Geometry check sheet. Reference: the model listing, model coordinates, mm. Face numbers are marked on the shaded views. A direction names the side the tool comes from. Round coordinates to 2 decimals unless told otherwise and drop trailing zeros. Order: outer loops, then holes, each group sorted by start corner. A loop starts at its lowest first (then second) coordinate and runs counter-clockwise, first axis right, second up.
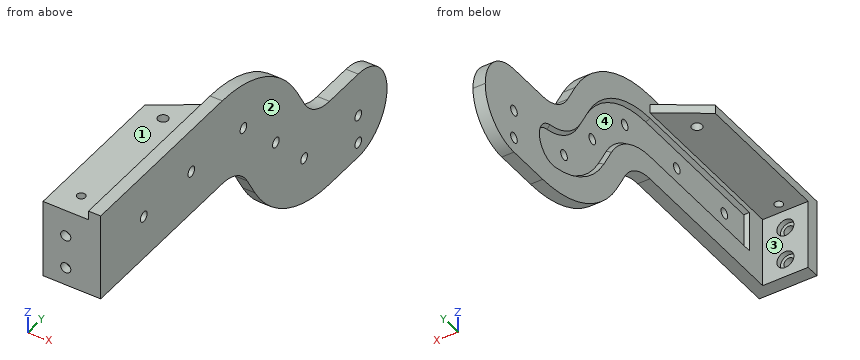
```python
from build123d import *

# Parameters (mm, degrees)
SKETCH_2_W                = 3.6
SKETCH_2_H                = 26
SKETCH_3_W                = 17
SKETCH_3_H                = 33
EXTRUDE_1_DEPTH           = 4
RIB_START                 = -1.3
RIB_1_DEPTH               = 2.6
SKETCH_5_R                = 1.5
SKETCH_5_R_2              = 1.224086187
CUT_EXTRUDE_1_DEPTH       = 4
CUT_EXTRUDE_2_DEPTH       = 4
SKETCH_7_R                = 1.5
CUT_EXTRUDE_3_DEPTH       = 4
CUT_EXTRUDE_4_DEPTH       = 1.2
CUT_EXTRUDE_4_DRAFT       = -30
HOLE_WIZARD_1_D           = 3
HOLE_WIZARD_1_CBORE_D     = 5
HOLE_WIZARD_1_CBORE_DEPTH = 1.6
CUT_EXTRUDE_6_DEPTH       = 135.185107528
SKETCH_25_R               = 1.5
CUT_EXTRUDE_8_DEPTH       = 139.143340278


# Read off the part's stored shape, not the designer's step: 筋1
with BuildPart() as part:
    # 扫描1: sweep along a path in 草图1
    with BuildLine(Plane(origin=(0, 0, 0), x_dir=(0, 0, -1), z_dir=(1, 0, 0))) as sweep_1_path:
        Line((0, 0), (0, 55))
        ThreePointArc((0, 55), (3.483339502, 68), (13, 77.516660498))
        Line((13, 77.516660498), (19, 80.980762114))
        ThreePointArc((19, 80.980762114), (28.516660498, 90.497422612), (32, 103.497422612))
        Line((32, 103.497422612), (32, 129.497422612))
    # 草图2 → 扫描1 (sweep)
    with BuildSketch(Plane(origin=(0, 0, 0), x_dir=(1, 0, 0), z_dir=(0, 1, 0))):
        Rectangle(SKETCH_2_W, SKETCH_2_H)
    sweep(path=sweep_1_path.line)

    # 草图3 → 凸台-拉伸1 (add)
    with BuildSketch(Plane.XZ):
        with Locations((-6.7, 3.5)):
            Rectangle(SKETCH_3_W, SKETCH_3_H)
    extrude(amount=-EXTRUDE_1_DEPTH)

    # 筋1 outline → 筋1 (add)
    with BuildSketch(Plane.XY.offset(9).offset(RIB_START)):
        Polygon((-1.8, 55), (-15.2, 46), (-15.2, 4), (-1.8, 4), align=None)
    extrude(amount=RIB_1_DEPTH)

    # 草图5 → 切除-拉伸1 (cut)
    with BuildSketch(Plane.XY.offset(10.3)):
        with Locations((-8.5, 44)):
            Circle(SKETCH_5_R)
        with Locations((-8.5, 7)):
            Circle(SKETCH_5_R_2)
    extrude(amount=-CUT_EXTRUDE_1_DEPTH, mode=Mode.SUBTRACT)

    # 草图6 → 切除-拉伸2 (cut)
    with BuildSketch(Plane.ZY.offset(1.8)):
        with BuildLine():
            Line((-45, 129.497422612), (-45, 116.497422612))
            ThreePointArc((-45, 116.497422612), (-41.192388155, 125.689810767), (-32, 129.497422612))
            Line((-32, 129.497422612), (-45, 129.497422612))
        make_face()
        with BuildLine():
            ThreePointArc((-32, 129.497422612), (-22.807611845, 125.689810767), (-19, 116.497422612))
            Line((-19, 116.497422612), (-19, 129.497422612))
            Line((-19, 129.497422612), (-32, 129.497422612))
        make_face()
    extrude(amount=-CUT_EXTRUDE_2_DEPTH, mode=Mode.SUBTRACT)

    # 草图7 → 切除-拉伸3 (cut)
    with BuildSketch(Plane(origin=(1.8, 0, 0), x_dir=(0, 0, -1), z_dir=(1, 0, 0))):
        with Locations((32, 116.497422612)):
            Circle(SKETCH_7_R)
        with Locations((40.5, 116.497422612)):
            Circle(SKETCH_7_R)
    extrude(amount=-CUT_EXTRUDE_3_DEPTH, mode=Mode.SUBTRACT)


with BuildPart() as cut_extrude_4_tool:
    # 草图8 → 切除-拉伸4 (with draft: the straight prism first)
    with BuildSketch(Plane.ZY.offset(1.8)):
        with BuildLine():
            Line((6, 10), (6, 55))
            ThreePointArc((6, 55), (1.712812921, 71), (-10, 82.712812921))
            Line((-10, 82.712812921), (-16, 86.176914536))
            ThreePointArc((-16, 86.176914536), (-22.383040886, 92.025893885), (-25.69615506, 100.024459059))
            ThreePointArc((-25.69615506, 100.024459059), (-32.646890644, 104.891416511), (-37.513848096, 97.940680927))
            ThreePointArc((-37.513848096, 97.940680927), (-32.212865417, 85.142976649), (-22, 75.784609691))
            Line((-22, 75.784609691), (-16, 72.320508076))
            ThreePointArc((-16, 72.320508076), (-8.679491924, 65), (-6, 55))
            Line((-6, 55), (-6, 10))
            Line((-6, 10), (6, 10))
        make_face()
    extrude(amount=-CUT_EXTRUDE_4_DEPTH)
    # 切除-拉伸4: the draft: its side faces are tilted about the plane it starts from
    cut_extrude_4_sides = [cut_extrude_4_tool.faces().sort_by_distance(p)[0] for p in [
        (-1.2, 32.5, 6),
        (-1.2, 71, 1.712812921),
        (-1.2, 84.444863729, -13),
        (-1.2, 92.025893885, -22.383040886),
        (-1.2, 104.891416511, -32.646890644),
        (-1.2, 85.142976649, -32.212865417),
        (-1.2, 74.052558883, -19),
        (-1.2, 65, -8.679491924),
        (-1.2, 32.5, -6),
        (-1.2, 10, 0),
    ]]
    draft(cut_extrude_4_sides, Plane.ZY.offset(1.8), CUT_EXTRUDE_4_DRAFT)


with BuildPart() as part_1:
    add(part.part)

    # 切除-拉伸4: cut by cut_extrude_4_tool
    add(cut_extrude_4_tool.part, mode=Mode.SUBTRACT)

    # 孔1 (through all)
    with Locations(Plane(origin=(0, 4, 0), x_dir=(1, 0, 0), z_dir=(0, 1, 0))):
        with Locations((-8.5, 7.65), (-8.5, -2.35)):
            CounterBoreHole(HOLE_WIZARD_1_D / 2, HOLE_WIZARD_1_CBORE_D / 2, HOLE_WIZARD_1_CBORE_DEPTH)

    # 草图18 → 切除-拉伸6 (cut, through all)
    with BuildSketch(Plane(origin=(0, 4, 0), x_dir=(1, 0, 0), z_dir=(0, 1, 0))):
        Polygon((-1.8, -13), (-1.8, -10.3), (-15.2, -10.3), (-15.2, -20), (1.8, -20), (1.8, -13), align=None)
    extrude(amount=-CUT_EXTRUDE_6_DEPTH, mode=Mode.SUBTRACT)

    # 草图25 → 切除-拉伸8 (cut, through all)
    with BuildSketch(Plane(origin=(1.8, 0, 0), x_dir=(0, 0, -1), z_dir=(1, 0, 0))):
        with Locations((0, 19.490691587)):
            Circle(SKETCH_25_R)
    cut_extrude_8 = extrude(amount=-CUT_EXTRUDE_8_DEPTH, mode=Mode.SUBTRACT)

    # 草图阵列1: 切除-拉伸8 at 4 more places
    with Locations((0, 21.499351, 0), (0, 45.068964, -1.821229), (0, 72.524124, -29.327017), (0, 59.75802, -16)):
        add(cut_extrude_8, mode=Mode.SUBTRACT)


solid = part_1.part
```
(1) Depth check by flat-ended pin: P1, Ø4, axis at x = -9, z = 3, coming from the +Y side; P2, Ø4, axis at x = -8.5, z = -7.65, coming from the -Y side; P3, Ø8.5, axis at x = -9.5, y = 39, coming from the -Z side; P4, Ø6.5, axis at x = -9, y = 33, coming from the +Z side. Enter the tip coordinate at first touch or a pass-through.
Returned:
P1: stops at y = 4
P2: stops at y = 0
P3: stops at z = 7.7
P4: stops at z = 10.3
(2) Sectioned sample at B-B, the plane x = -8.5. Give the number of separate pieces and of enclosed holes in the cut face, and give its area (3 significant figures).
Returned:
separate pieces: 5
enclosed holes: 0
area: 170 mm2
(3) Sectioned sample at C-C, the plane y = 107. Record the cut outline in (x, z), and give its area (3 significant figures).
Returned:
outline: (-1.8, -45) - (1.8, -45) - (1.8, -19) - (-1.8, -19) - close
area: 93.6 mm2
(4) Sectioned sample at A-A, the plane y = 7. Record the cut outline in (x, z).
Returned:
outline: (-15.2, 7.7) - (-9.72, 7.7) - (-9.72, 10.3) - (-15.2, 10.3) - close; (-7.28, 7.7) - (-1.8, 7.7) - (-1.8, -13) - (1.8, -13) - (1.8, 13) - (-1.8, 13) - (-1.8, 10.3) - (-7.28, 10.3) - close
(5) Set-up check for the marked faces 1, 2, 3 and 4: record each of +Z, -Z, +X, -X, +Y, -Y from which the full face is reachable in a straight line by a thin tool's end or side.
Returned:
face 1: +Z, -X, +Y, -Y
face 2: +Z, -Z, +X, +Y, -Y
face 3: -Z, -X, +Y
face 4: -X
(6) Material ranges on line 1 (Z direction, x = -8.5, y = 3.55); line 2 (Z direction, x = -8.5, y = 1.4); line 3 (Y direction, x = -8.5, z = 8.8), recorded low to high.
Returned:
line 1: z = -13 to -10.15, -5.15 to -0.15, 4.85 to 10.3
line 2: z = -13 to -9.15, -6.15 to 0.85, 3.85 to 10.3
line 3: y = 0 to 5.78, 8.22 to 42.5, 45.5 to 50.5
